```python
from build123d import *

# Parameters (mm, degrees)
PAD_DEPTH = 2.5


with BuildPart() as part:
    # Sketch → Pad (new body, symmetric)
    with BuildSketch(Plane.XY):
        with BuildLine():
            Line((75.5, 82), (75.5, -82))
            Line((75.5, -82), (55.5, -82))
            Line((55.5, -82), (55.5, -77))
            Line((55.5, -77), (-55.5, -77))
            Line((-55.5, -77), (-55.5, -82))
            Line((-55.5, -82), (-75.5, -82))
            Line((-75.5, -82), (-75.5, -6))
            Line((-5.5, -6), (-75.5, -6))
            ThreePointArc((-5.5, -6), (13.5, 13), (-5.5, 32))
            Line((-75.5, 32), (-5.5, 32))
            Line((-75.5, 32), (-75.5, 82))
            Line((-75.5, 82), (-55.5, 82))
            Line((-55.5, 82), (-55.5, 77))
            Line((-55.5, 77), (55.5, 77))
            Line((55.5, 77), (55.5, 82))
            Line((55.5, 82), (75.5, 82))
        make_face()
    extrude(amount=PAD_DEPTH, both=True)


solid = part.part
```
Design review of the part built by this model. Coordinates are the model's own, in mm. A direction names the side the tool comes from. Coordinates: 2 decimals unless noted, no trailing zeros. Order: outer loops, then holes, each group sorted by start corner. A loop starts at its lowest first (then second) coordinate and runs counter-clockwise, first axis right, second up. Notation, with made-up numbers: (-28, 82.5) - (-19, 82.5) arc R18 ccw to (-19, 89.5) - close; hole circle Ø5 at (-16.5, 25.5). An arc over 180 degrees is marked (long way). Answer in a Markdown table with one row per item.
(1) Wall thickness on line 1 along Y through (x, z) = (-52, 1.8); line 2 along Y through (x, z) = (46, -0.65); line 3 along X through (y, z) = (13, -2): over which ranges is each line inside the solid? List them lowest first. Write a range as from..to.
Checked values:
| item | result |
|---|---|
| line 1 | -77..-6, 32..77 |
| line 2 | -77..77 |
| line 3 | 13.5..75.5 |
(2) Consider section A-A on x = -48.5. State the section outline as (y, z) points, plus the area to 3 significant figures.
Checked values:
| item | result |
|---|---|
| outline | (-77, -2.5) - (-6, -2.5) - (-6, 2.5) - (-77, 2.5) - close; (32, -2.5) - (77, -2.5) - (77, 2.5) - (32, 2.5) - close |
| area | 580 mm^2 |
(3) The part is to be moulded in two halves that separate along Y. For faces 1 (the flat face through (55.5, -80, 0)), 2 (the flat face through (66, -82, 0)), 3 (the flat face through (-41, 32, 0)), say which applies: released by +Y, released by -Y, zero draft, split by the parting line, or undercut.
Checked values:
| item | result |
|---|---|
| face 1 | zero draft |
| face 2 | released by -Y |
| face 3 | undercut |
(4) Consider section B-B on z = -0.3. State the section outline as (x, y) points, plus the area to 3 significant figures.
Checked values:
| item | result |
|---|---|
| outline | (-75.5, -82) - (-55.5, -82) - (-55.5, -77) - (55.5, -77) - (55.5, -82) - (75.5, -82) - (75.5, 82) - (55.5, 82) - (55.5, 77) - (-55.5, 77) - (-55.5, 82) - (-75.5, 82) - (-75.5, 32) - (-5.5, 32) arc R19 cw to (-5.5, -6) - (-75.5, -6) - close |
| area | 20,400 mm^2 |
(5) Consider section C-C on y = 13. State the section outline as (x, z) points.
Checked values:
| item | result |
|---|---|
| outline | (13.5, -2.5) - (75.5, -2.5) - (75.5, 2.5) - (13.5, 2.5) - close |
(6) For faces 4 (the flat face through (-55.5, -79, 0)), 5 (the flat face through (-1, 77, 0)), 6 (the flat face through (-40, -6, 0)), 7 (the flat face through (65, 82, 0)), 8 (the flat face through (18, 1, 2.5)), list the 3-axis set-ups (+Z, -Z, +X, -X, +Y, -Y) from which the entire face can be reached by the end or side of a thin tool; tool diameter is ignored.
Checked values:
| item | result |
|---|---|
| face 4 | +Z, -Z, -Y |
| face 5 | +Z, -Z, +Y |
| face 6 | +Z, -Z, -X |
| face 7 | +Z, -Z, +X, -X, +Y |
| face 8 | +Z, +X, -X, +Y, -Y |
(7) Clearance check with flat-ended pins moving along their axes: pin 1 (2.5 mm diameter, centred on x = 2.5, z = 0.5, fed in from +Y); pin 2 (2.5 mm diameter, centred on x = 5.5, z = 0, fed in from -Y). State where each tip first meets the part, or that it passes through.
Checked values:
| item | result |
|---|---|
| pin 1 | y = 77 |
| pin 2 | y = -77 |
(8) Consider section D-D on x = 24. State the section outline as (y, z) points.
Checked values:
| item | result |
|---|---|
| outline | (-77, -2.5) - (77, -2.5) - (77, 2.5) - (-77, 2.5) - close |
